```python
from build123d import *

# Parameters (mm, degrees)
BOSS_EXTRUDE1_DEPTH = 4
FILLET1_R           = 5
SKETCH2_R           = 1.5
CUT_EXTRUDE1_DEPTH  = 17.091809531
CIRPATTERN1_COUNT   = 6


with BuildPart() as part:
    # Sketch1 → Boss-Extrude1 (new body)
    with BuildSketch(Plane.XY):
        Polygon((6.109123402, -10.581312122), (12.218246804, 0), (6.109123402, 10.581312122), (-6.109123402, 10.581312122), (-12.218246804, 0), (-6.109123402, -10.581312122), align=None)
    extrude(amount=BOSS_EXTRUDE1_DEPTH)

    # Fillet1
    fillet1_edges = [part.edges().sort_by_distance(p)[0] for p in [
        (-6.109123402, -10.581312122, 2),
        (-12.218246804, 0, 2),
        (-6.109123402, 10.581312122, 2),
        (6.109123402, 10.581312122, 2),
        (12.218246804, 0, 2),
        (6.109123402, -10.581312122, 2),
    ]]
    fillet(fillet1_edges, radius=FILLET1_R)

    # Sketch2 → Cut-Extrude1 (cut, through all)
    with BuildSketch(Plane.XY.offset(4)):
        with Locations((-4.111186028, -7.12078308)):
            Circle(SKETCH2_R)
    cut_extrude1 = extrude(amount=-CUT_EXTRUDE1_DEPTH, mode=Mode.SUBTRACT)

    # CirPattern1: Cut-Extrude1 ×6 about axis
    cirpattern1_axis = Axis((0, 0, 0), (0, 0, 1))
    for i in range(1, CIRPATTERN1_COUNT):
        add(cut_extrude1.rotate(cirpattern1_axis, i * 360 / CIRPATTERN1_COUNT), mode=Mode.SUBTRACT)


solid = part.part
```
Can you work these out from the model? Positions are in its coordinate system, mm. Round coordinates to 2 decimals unless told otherwise and drop trailing zeros. Loops run counter-clockwise (first coordinate to the right, second up) from the corner with the lowest first, then second, coordinate; pieces in that order, holes last. Notation, with made-up numbers: (78, 38.5) -> (91, 38.5) arc R12 ccw to (91, 42.5) -> close; hole circle Ø4 at (84, -36). An arc over 180 degrees is marked (long way). One line per item, written item: value. Start each with the question number.
1. If I drill on probe 1 along Y at (x, z) = (-4, 1); probe 2 along Y at (x, z) = (-3.75, 0.75); probe 3 along X at (y, z) = (8.25, 1.75), over which ranges is the centre line in solid material (lowest first)?
2. If we mould it in two halves opening along X, with no side actions, what happens to faces 1 (the flat face through (9.14, -5.33, 1.97)), 2 (the flat face through (-9.14, 5.33, 1.97)), 3 (the cylindrical face through (2.726, -6.546, 2.028)), 4 (the cylindrical face through (-2.726, 6.546, 2.028))? For each: pulls with the +X half, pulls with the -X half, needs draft (parallel to the pull), parting line crosses it, or undercut.
3. If we section it at B-B, the plane z = 1.75: Write out the boundary of the cut face in (x, y).
4. If we section it at C-C, the plane x = -9: Write out the boundary of the cut face in (y, z), then the cut area to 3 significant figures.
5. If we section it at D-D, the plane y = -3.25: Write out the boundary of the cut face in (x, z), then the cut area to 3 significant figures.
6. For pin 1 (3.5 mm diameter, centred on x = 4.11, y = 7.12, fed in from -Z); pin 2 (2.5 mm diameter, centred on x = 8.22, y = 0, fed in from -Z); pin 3 (1 mm diameter, centred on y = -5, z = 0.5, fed in from +X); pin 4 (2 mm diameter, centred on y = -1.5, z = 2.5, fed in from -X), each with a flat end and sliding along its axis, tell me the tip position at first contact or that it passes through.
7. If we section it at A-A, the plane y = 0: Write out the boundary of the cut face in (x, z).
Calculated:
1. probe 1: y = -10.52 to -8.62, -5.62 to 5.62, 8.62 to 10.52
1. probe 2: y = -10.55 to -8.58, -5.66 to 5.66, 8.58 to 10.55
1. probe 3: x = -7.45 to -5.1, -3.12 to 3.12, 5.1 to 7.45
2. face 1: pulls with the +X half
2. face 2: pulls with the -X half
2. face 3: undercut
2. face 4: undercut
3. outline: (-10.77, -2.5) -> (-7.55, -8.08) arc R5 ccw to (-3.22, -10.58) -> (3.22, -10.58) arc R5 ccw to (7.55, -8.08) -> (10.77, -2.5) arc R5 ccw to (10.77, 2.5) -> (7.55, 8.08) arc R5 ccw to (3.22, 10.58) -> (-3.22, 10.58) arc R5 ccw to (-7.55, 8.08) -> (-10.77, 2.5) arc R5 ccw to start; hole circle Ø3 at (-8.22, 0); hole circle Ø3 at (-4.11, -7.12); hole circle Ø3 at (-4.11, 7.12); hole circle Ø3 at (4.11, -7.12); hole circle Ø3 at (4.11, 7.12); hole circle Ø3 at (8.22, 0)
4. outline: (-5.57, 0) -> (-1.28, 0) -> (-1.28, 4) -> (-5.57, 4) -> close; (1.28, 0) -> (5.57, 0) -> (5.57, 4) -> (1.28, 4) -> close
4. area: 34.3 mm²
5. outline: (-10.34, 0) -> (10.34, 0) -> (10.34, 4) -> (-10.34, 4) -> close
5. area: 82.7 mm²
6. pin 1: stops at z = 0
6. pin 2: passes through
6. pin 3: stops at x = 9.62
6. pin 4: stops at x = -11.42
7. outline: (-11.44, 0) -> (-9.72, 0) -> (-9.72, 4) -> (-11.44, 4) -> close; (-6.72, 0) -> (6.72, 0) -> (6.72, 4) -> (-6.72, 4) -> close; (9.72, 0) -> (11.44, 0) -> (11.44, 4) -> (9.72, 4) -> close
